from build123d import *

# Parameters (mm, degrees)
PAD004_DEPTH        = 16
FILLET003_R         = 2.5
HOLE003_D           = 4.5
HOLE003_CBORE_D     = 5.6
HOLE003_CBORE_DEPTH = 4.4
HOLE004_D           = 7.1
HOLE004_CBORE_D     = 11.36
HOLE004_CBORE_DEPTH = 15.89
CHAMFER006_SIZE     = 0.4


with BuildPart() as part:
    # Sketch017 → Pad004 (new body)
    with BuildSketch(Plane.XY):
        with BuildLine():
            Line((9.367497, 7.5), (21, 7.5))
            Line((21, 7.5), (21, -7.5))
            Line((21, -7.5), (9.367497, -7.5))
            ThreePointArc((0, -12), (5.196152, -10.816654), (9.367497, -7.5))
            Line((0, -12), (-21, -12))
            Line((-21, -12), (-21, -8))
            Line((-21, -8), (-4.123106, -8))
            ThreePointArc((-4.123106, -8), (9, 0), (-4.123106, 8))
            Line((-21, 8), (-4.123106, 8))
            Line((-21, 11), (-21, 8))
            Line((-4.795832, 11), (-21, 11))
            ThreePointArc((9.367497, 7.5), (2.878807, 11.649569), (-4.795832, 11))
        make_face()
    extrude(amount=PAD004_DEPTH)

    # Fillet003
    fillet003_edges = [part.edges().sort_by_distance(p)[0] for p in [
        (-21, -10, 16),
        (-21, 9.5, 16),
        (-21, 9.5, 0),
        (-21, -10, 0),
    ]]
    fillet(fillet003_edges, radius=FILLET003_R)

    # Hole003 (through all)
    with Locations(Plane.XZ.offset(12)):
        with Locations((-13, 8)):
            CounterBoreHole(HOLE003_D / 2, HOLE003_CBORE_D / 2, HOLE003_CBORE_DEPTH)

    # Hole004 (through all)
    with Locations(Plane(origin=(0, 0, 0), x_dir=(0, 1, 0), z_dir=(-1, 0, 0))):
        with Locations((0, -8)):
            CounterBoreHole(HOLE004_D / 2, HOLE004_CBORE_D / 2, HOLE004_CBORE_DEPTH)

    # Chamfer006
    chamfer006_edges = [part.edges().sort_by_distance(p)[0] for p in [
        (21, 0, 16),
        (15.183748, 7.5, 16),
        (15.183748, -7.5, 16),
        (5.196152, -10.816654, 16),
        (9, 0, 16),
        (2.878807, 11.649569, 16),
        (-11.647916, 11, 16),
        (-11.311553, 8, 16),
        (-11.311553, -8, 16),
        (-9.25, -12, 16),
        (15.183748, 7.5, 0),
        (21, 0, 0),
        (2.878807, 11.649569, 0),
        (9, 0, 0),
        (-11.647916, 11, 0),
        (-11.311553, 8, 0),
        (15.183748, -7.5, 0),
        (5.196152, -10.816654, 0),
        (-9.25, -12, 0),
        (-11.311553, -8, 0),
    ]]
    chamfer(chamfer006_edges, length=CHAMFER006_SIZE)


solid = part.part
Geometry: final body of the model. Coordinates: model frame, mm. A direction names the side the tool comes from. Coordinates: 2 decimals unless noted, no trailing zeros. Order: outer loops, then holes, each group sorted by start corner. A loop starts at its lowest first (then second) coordinate and runs counter-clockwise, first axis right, second up. Notation, with made-up numbers: (6, 52.25) - (43, 52.25) arc R21 ccw to (43, 65.25) - close; hole circle Ø3 at (-4, -27). An arc over 180 degrees is marked (long way). Use one line per item in the form item = value.
1) Section A-A (x = -6). Return loops of the section in (y, z), then the cut area to 3 significant figures.
Solutions:
outline = (-12, 0.4) - (-11.6, 0) - (-8.4, 0) - (-8, 0.4) - (-8, 15.6) - (-8.4, 16) - (-11.6, 16) - (-12, 15.6) - close; (8, 0.4) - (8.4, 0) - (10.6, 0) - (11, 0.4) - (11, 15.6) - (10.6, 16) - (8.4, 16) - (8, 15.6) - close
area = 111 mm^2
2) Set-up query: faces 1 (the face through (-20.044, 8.108, 0.921)), 2 (the face through (-13.607, -10.028, 5.267)), 3 (the face through (12.363, 5.247, 10.175)), 4 (the face through (15, 7.5, 8)). Return all of +Z, -Z, +X, -X, +Y, -Y with unobstructed straight access to the full face (end or side cutting, diameter ignored); none if empty.
Solutions:
face_1 = -Z, -X
face_2 = -Y
face_3 = -X
face_4 = +Z, -Z, +X, +Y
3) Section B-B (z = 8). State how many separate pieces and enclosed holes the cut face has, then the cut area to 3 significant figures.
Solutions:
separate_pieces = 4
enclosed_holes = 0
area = 233 mm^2
4) Ray query, L1, parallel to Z at x = 19.2, y = 0; L2, parallel to Y at x = -11, z = 14.75; L3, parallel to Z at x = 14, y = 0. Return the intervals inside material, ascending.
Solutions:
L1 = 0 to 4.45, 11.55 to 16
L2 = -12 to -8, 8 to 11
L3 = 0 to 2.32, 13.68 to 16
5) Mould query, pull axis Z, two halves, no side actions, for faces 5 (the face through (-20.044, 10.892, 15.079)), 6 (the face through (-20.079, 10.892, 0.956)), 7 (the face through (15.89, 0, 12)). Classes: +Z half, -Z half, draft (parallel to the pull), parting line (faces both ways), or undercut.
Solutions:
face_5 = +Z half
face_6 = -Z half
face_7 = undercut
6) Section D-D (x = -13). Return loops of the section in (y, z), then the cut area to 3 significant figures.
Solutions:
outline = (-12, 0.4) - (-11.6, 0) - (-8.4, 0) - (-8, 0.4) - (-8, 5.2) - (-12, 5.2) - close; (-12, 10.8) - (-8, 10.8) - (-8, 15.6) - (-8.4, 16) - (-11.6, 16) - (-12, 15.6) - close; (8, 0.4) - (8.4, 0) - (10.6, 0) - (11, 0.4) - (11, 5.75) - (8, 5.75) - close; (8, 10.25) - (11, 10.25) - (11, 15.6) - (10.6, 16) - (8.4, 16) - (8, 15.6) - close
area = 75.5 mm^2
7) Section C-C (y = 0). Return loops of the section in (x, z).
Solutions:
outline = (9, 0.4) - (9.4, 0) - (20.6, 0) - (21, 0.4) - (21, 4.45) - (15.89, 4.45) - (15.89, 2.32) - (9, 2.32) - close; (9, 13.68) - (15.89, 13.68) - (15.89, 11.55) - (21, 11.55) - (21, 15.6) - (20.6, 16) - (9.4, 16) - (9, 15.6) - close
8) Pin query (flat end, axial travel): pin 1 (9.5 mm diameter, centred on x = 16.5, z = 8, fed in from -Y); pin 2 (1.5 mm diameter, centred on x = 3, z = 10, fed in from -Y); pin 3 (5.5 mm diameter, centred on y = 1.5, z = 9, fed in from -X); pin 4 (8 mm diameter, centred on x = -2, y = -1, fed in from +Z). Return the tip coordinate at first contact, or that it passes through.
Solutions:
pin_1 = -7.5
pin_2 = -11.79
pin_3 = 15.89
pin_4 = through
